For this review, use the dimensioned drawing (mm, ordinates from the lowest corner) and the shaded views. Round coordinates to 2 decimals unless told otherwise and drop trailing zeros. Order: outer loops, then holes, each group sorted by start corner. A loop starts at its lowest first (then second) coordinate and runs counter-clockwise, first axis right, second up. Notation, with made-up numbers: M -6,12.25 L 4,12.25 A17 ccw 4,16.25 Z; hole C 36.25,-23.75 d2. An arc over 180 degrees is marked long. Put each result on its own line as item: value.
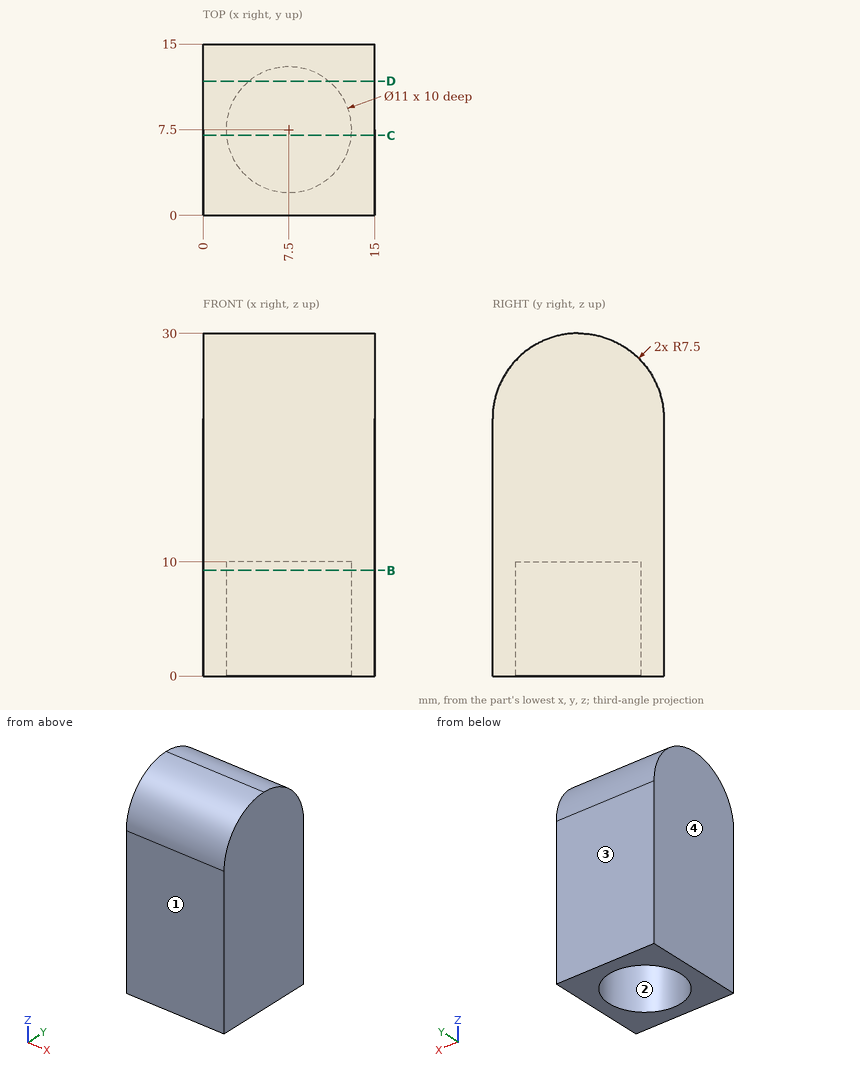
(1) Draft analysis for pull direction Y (two halves, no side actions). For the marked faces 1, 2, 3 and 4, state which applies: released by +Y, released by -Y, zero draft, split by the parting line, or undercut.
A:
face 1: released by -Y
face 2: undercut
face 3: released by +Y
face 4: zero draft
(2) Add section C-C on y = 7. Give the boundary of the cut face in (x, z).
A:
outline: M 0,0 L 2.02,0 L 2.02,10 L 12.98,10 L 12.98,0 L 15,0 L 15,29.98 L 0,29.98 Z
(3) Add section D-D on y = 11.75. Give the boundary of the cut face in (x, z), then the cut area to 3 significant figures.
A:
outline: M 0,0 L 4.01,0 L 4.01,10 L 10.99,10 L 10.99,0 L 15,0 L 15,28.68 L 0,28.68 Z
area: 360 mm2
(4) Add section B-B on z = 9.25. Give the boundary of the cut face in (x, y).
A:
outline: M 0,0 L 15,0 L 15,15 L 0,15 Z; hole C 7.5,7.5 d11
(5) To check wall thickness, follow L1, parallel to Y at x = 7.5, z = 2.5; L2, parallel to X at y = 5.5, z = 3.5; L3, parallel to X at y = 4, z = 6.25. State the ranges of each line that lie inside material, in increasing order.
A:
L1: y = 0 to 2, 13 to 15
L2: x = 0 to 2.38, 12.62 to 15
L3: x = 0 to 3.26, 11.74 to 15
